Geometry: final body of the model. Coordinates: model frame, mm. A direction names the side the tool comes from. Give positions to 0.01 mm unless a question says otherwise; leave off trailing zeros. Loops run counter-clockwise (first coordinate to the right, second up) from the corner with the lowest first, then second, coordinate; pieces in that order, holes last.
from build123d import *

# Parameters (mm, degrees)
F0_W     = 49.022
F0_H     = 22.098
F1_DEPTH = 9.652
F3_DEPTH = 7.62
F4_SIZE  = 2.032


with BuildPart() as f1:
    # F0 (on Top) → F1 (new body)
    with BuildSketch(Plane.XY):
        Rectangle(F0_W, F0_H)
    extrude(amount=F1_DEPTH)

    # F2 (on face) → F3 (cut)
    with BuildSketch(Plane.XY.offset(9.652)):
        Polygon((22.479, 9.017), (-22.479, 9.017), (-22.479, 4.28625), (-22.479, -4.28625), (-22.479, -9.017), (22.479, -9.017), align=None)
    extrude(amount=-F3_DEPTH, mode=Mode.SUBTRACT)

    # F4
    f4_edges = [f1.edges().sort_by_distance(p)[0] for p in [
        (0, -11.049, 0),
        (24.511, 0, 0),
        (24.511, -11.049, 4.826),
        (24.511, 11.049, 4.826),
        (-24.511, 0, 0),
        (0, 11.049, 0),
        (-24.511, -11.049, 4.826),
        (-24.511, 11.049, 4.826),
    ]]
    chamfer(f4_edges, length=F4_SIZE)


solid = f1.part
Item 1: Section query B-B on y = 6.5. Return loops of the section in (x, z), plus the area to 3 significant figures.
Values follow:
outline: (-24.51, 2.03) - (-22.48, 0) - (22.48, 0) - (24.51, 2.03) - (24.51, 9.65) - (22.48, 9.65) - (22.48, 2.03) - (-22.48, 2.03) - (-22.48, 9.65) - (-24.51, 9.65) - close
area: 126 mm2
Item 2: Section query C-C on x = -15.5. Return loops of the section in (y, z).
Values follow:
outline: (-11.05, 2.03) - (-9.02, 0) - (9.02, 0) - (11.05, 2.03) - (11.05, 9.65) - (9.02, 9.65) - (9.02, 2.03) - (-9.02, 2.03) - (-9.02, 9.65) - (-11.05, 9.65) - close
Item 3: Ray query, probe 1 along X at (y, z) = (-5.5, 2.25); probe 2 along Y at (x, z) = (-16, 5.5); probe 3 along Z at (x, y) = (13.5, 1.75). Return the intervals inside material, ascending.
Values follow:
probe 1: x = -24.51 to -22.48, 22.48 to 24.51
probe 2: y = -11.05 to -9.02, 9.02 to 11.05
probe 3: z = 0 to 2.03
Item 4: Draft query along Y for faces 3 (the face through (0, -9.017, 6)), 4 (the face through (0, 9.017, 6)), 5 (the face through (-0.315, -10.019, 1.002)), 6 (the face through (23.51, -0.13, 1.03)). Return one class per face: +Y half, -Y half, draft (parallel to the pull), parting line (faces both ways), or undercut.
Values follow:
face 3: undercut
face 4: undercut
face 5: -Y half
face 6: draft
Item 5: Set-up query: faces 1 (the face through (-22.479, 0, 6)), 2 (the face through (-23.255, -9.631, 1.39)). Return all of +Z, -Z, +X, -X, +Y, -Y with unobstructed straight access to the full face (end or side cutting, diameter ignored); none if empty.
Values follow:
face 1: +Z
face 2: -Z, -X, -Y
Item 6: Section query D-D on z = 1.5. Return loops of the section in (x, y), plus the area to 3 significant figures.
Values follow:
outline: (-23.98, -9.02) - (-22.48, -10.52) - (22.48, -10.52) - (23.98, -9.02) - (23.98, 9.02) - (22.48, 10.52) - (-22.48, 10.52) - (-23.98, 9.02) - close
area: 1,000 mm2
Item 7: Section query A-A on z = 4. Return loops of the section in (x, y), plus the area to 3 significant figures.
Values follow:
outline: (-24.51, -9.02) - (-22.48, -11.05) - (22.48, -11.05) - (24.51, -9.02) - (24.51, 9.02) - (22.48, 11.05) - (-22.48, 11.05) - (-24.51, 9.02) - close; hole (-22.48, -9.02) - (22.48, -9.02) - (22.48, 9.02) - (-22.48, 9.02) - close
area: 264 mm2
Item 8: Pin query (flat end, axial travel): pin 1 (9 mm diameter, centred on x = 11, y = -4, fed in from +Z). Return the tip coordinate at first contact, or that it passes through.
Values follow:
pin 1: stops at z = 2.03
